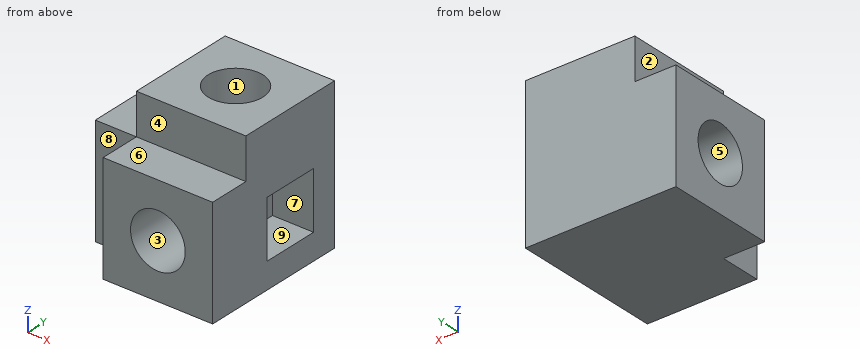
```python
from build123d import *

# Parameters (mm, degrees)
ESQUISSE2_W             = 80
ESQUISSE2_H             = 80
BOSS_EXTRU_1_DEPTH      = 80
ESQUISSE5_W             = 80
ESQUISSE5_H             = 80
BOSS_EXTRU_2_DEPTH      = 30
ESQUISSE6_W             = 80
ESQUISSE6_H             = 80
BOSS_EXTRU_3_DEPTH      = 30
ESQUISSE7_W             = 80
ESQUISSE7_H             = 80
BOSS_EXTRU_4_DEPTH      = 30
ESQUISSE8_R             = 20
ENL_V_MAT_EXTRU_1_DEPTH = 45
ESQUISSE9_R             = 20
ENL_V_MAT_EXTRU_2_DEPTH = 45
ESQUISSE10_R            = 20
ENL_V_MAT_EXTRU_3_DEPTH = 45
ESQUISSE11_W            = 42
ESQUISSE11_H            = 42
ENL_V_MAT_EXTRU_4_DEPTH = 30


with BuildPart() as part:
    # Esquisse2 → Boss.-Extru.1 (new body)
    with BuildSketch(Plane(origin=(0, 0, 0), x_dir=(1, 0, 0), z_dir=(0, 1, 0))):
        Rectangle(ESQUISSE2_W, ESQUISSE2_H)
    extrude(amount=BOSS_EXTRU_1_DEPTH)

    # Esquisse5 → Boss.-Extru.2 (add)
    with BuildSketch(Plane.ZY.offset(40)):
        with Locations((0, 40)):
            Rectangle(ESQUISSE5_W, ESQUISSE5_H)
    extrude(amount=BOSS_EXTRU_2_DEPTH)

    # Esquisse6 → Boss.-Extru.3 (add)
    with BuildSketch(Plane.XY.offset(40)):
        with Locations((0, 40)):
            Rectangle(ESQUISSE6_W, ESQUISSE6_H)
    extrude(amount=BOSS_EXTRU_3_DEPTH)

    # Esquisse7 → Boss.-Extru.4 (add)
    with BuildSketch(Plane.XZ):
        Rectangle(ESQUISSE7_W, ESQUISSE7_H)
    extrude(amount=BOSS_EXTRU_4_DEPTH)

    # Esquisse8 → Enlèv. mat.-Extru.1 (cut)
    with BuildSketch(Plane.ZY.offset(70)):
        with Locations((0, 40)):
            Circle(ESQUISSE8_R)
    extrude(amount=-ENL_V_MAT_EXTRU_1_DEPTH, mode=Mode.SUBTRACT)

    # Esquisse9 → Enlèv. mat.-Extru.2 (cut)
    with BuildSketch(Plane.XY.offset(70)):
        with Locations((0, 40)):
            Circle(ESQUISSE9_R)
    extrude(amount=-ENL_V_MAT_EXTRU_2_DEPTH, mode=Mode.SUBTRACT)

    # Esquisse10 → Enlèv. mat.-Extru.3 (cut)
    with BuildSketch(Plane.XZ.offset(30)):
        with Locations(Location((0, 0, 0), (0, 0, 270))):
            Circle(ESQUISSE10_R)
    extrude(amount=-ENL_V_MAT_EXTRU_3_DEPTH, mode=Mode.SUBTRACT)

    # Esquisse11 → Enlèv. mat.-Extru.4 (cut)
    with BuildSketch(Plane(origin=(40, 0, 0), x_dir=(0, 0, -1), z_dir=(1, 0, 0))):
        with Locations((0, 40)):
            Rectangle(ESQUISSE11_W, ESQUISSE11_H)
    extrude(amount=-ENL_V_MAT_EXTRU_4_DEPTH, mode=Mode.SUBTRACT)


solid = part.part
```
The model under review builds one solid part; all positions refer to its coordinate system, in mm. Face numbers are marked on the shaded views. A direction names the side the tool comes from. Round coordinates to 2 decimals unless told otherwise and drop trailing zeros. Loops run counter-clockwise (first coordinate to the right, second up) from the corner with the lowest first, then second, coordinate; pieces in that order, holes last. Notation, with made-up numbers: M 58,79 L 81,79 A10 cw 81,90 Z; hole C 3,73.25 d6. An arc over 180 degrees is marked long. Answer as a JSON object with one key per item and string values.
(1) Draft analysis for pull direction Y (two halves, no side actions). For the marked faces 6, 7, 8 and 9, state which applies: released by +Y, released by -Y, zero draft, split by the parting line, or undercut.
Resolved:
{"face 6": "zero draft", "face 7": "undercut", "face 8": "released by -Y", "face 9": "undercut"}
(2) To check wall thickness, follow line 1 along Y through (x, z) = (0, 42.5); line 2 along Y through (x, z) = (30.5, 6); line 3 along Z through (x, y) = (-36, -14). State the ranges of each line that lie inside material, in increasing order.
Resolved:
{"line 1": "0 to 20, 60 to 80", "line 2": "-30 to 19, 61 to 80", "line 3": "-40 to 40"}
(3) Take a section at B-B on z = 44. Give the boundary of the cut face in (x, y), and give its area (3 significant figures).
Resolved:
{"outline": "M -40,0 L 40,0 L 40,80 L -40,80 Z; hole C 0,40 d40", "area": "5,140 mm²"}
(4) Clearance check with flat-ended pins moving along their axes: P1, Ø1, axis at x = 15.5, z = -5.5, coming from the -Y side; P2, Ø9, axis at y = 46, z = 59.5, coming from the -X side; P3, Ø12, axis at y = 41, z = -8.5, coming from the -X side. State where each tip first meets the part, or that it passes through.
Resolved:
{"P1": "y = 15", "P2": "x = -40", "P3": "x = -25"}
(5) Take a section at D-D on z = 0. Give the boundary of the cut face in (x, y).
Resolved:
{"outline": "M -70,0 L -40,0 L -40,-30 L -20,-30 L -20,15 L 20,15 L 20,-30 L 40,-30 L 40,19 L 10,19 L 10,61 L 40,61 L 40,80 L -70,80 L -70,60 L -25,60 L -25,20 L -70,20 Z"}
(6) Take a section at C-C on y = 56. Give the boundary of the cut face in (x, z), and give its area (3 significant figures).
Resolved:
{"outline": "M -70,-40 L 40,-40 L 40,-21 L 10,-21 L 10,21 L 40,21 L 40,70 L 12,70 L 12,25 L -12,25 L -12,70 L -40,70 L -40,40 L -70,40 L -70,12 L -25,12 L -25,-12 L -70,-12 Z", "area": "7,780 mm²"}
(7) Tool access review of the marked faces 1, 2, 3, 4 and 5: name each direction out of +Z, -Z, +X, -X, +Y, -Y from which nothing blocks a thin tool from reaching the whole face with its end or side.
Resolved:
{"face 1": "+Z", "face 2": "+Z, -X, +Y, -Y", "face 3": "-Y", "face 4": "+Z, +X, -X, -Y", "face 5": "-X"}
(8) Take a section at A-A on x = 33.5. Give the boundary of the cut face in (y, z), and give its area (3 significant figures).
Resolved:
{"outline": "M -30,-40 L 80,-40 L 80,70 L 0,70 L 0,40 L -30,40 Z; hole M 19,-21 L 61,-21 L 61,21 L 19,21 Z", "area": "9,440 mm²"}
